The drawing under review shows one solid part. Ordinate dimensions are in mm from its lowest x, y, z. Coordinates: 2 decimals unless noted, no trailing zeros. Write each loop counter-clockwise with the first axis right and the second up, starting at its lowest first coordinate (ties: lowest second). Pieces come first, ordered by that corner, then holes. Notation, with made-up numbers: (-23, 88) - (-12, 88) arc R29 cw to (-12, 124) - close; hole circle Ø11 at (-34.5, -16.5). An arc over 180 degrees is marked (long way). Use a Markdown table: item, result.
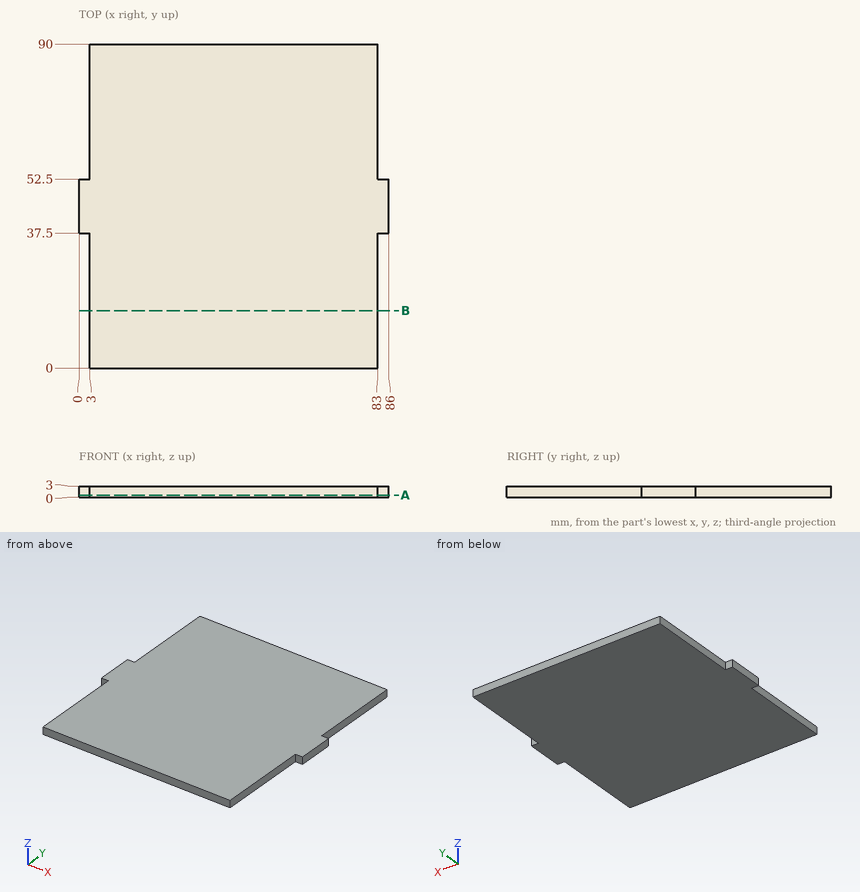
(1) Take a section at A-A on z = 0.55. Write out the cut boundary in (x, y), and give its area (3 significant figures).
Determined:
| item | result |
|---|---|
| outline | (0, 37.5) - (3, 37.5) - (3, 0) - (83, 0) - (83, 37.5) - (86, 37.5) - (86, 52.5) - (83, 52.5) - (83, 90) - (3, 90) - (3, 52.5) - (0, 52.5) - close |
| area | 7,290 mm2 |
(2) For L1, parallel to X at y = 18.5, z = 1.7, list the stretches that pass through material, from the lowest coordinate up. Write a range as from..to.
Determined:
| item | result |
|---|---|
| L1 | 3..83 |
(3) Take a section at B-B on y = 16. Write out the cut boundary in (x, z), and give its area (3 significant figures).
Determined:
| item | result |
|---|---|
| outline | (3, 0) - (83, 0) - (83, 3) - (3, 3) - close |
| area | 240 mm2 |
(4) For pin 1 (1.5 mm diameter, centred on x = 84, z = 1.5, fed in from +Y); pin 2 (0.9 mm diameter, centred on y = 76, z = 1.5, fed in from -X); pin 3 (1.5 mm diameter, centred on x = 2, z = 1.5, fed in from -Y), all flat-tipped, find the tip position at first contact; note any pin that passes through.
Determined:
| item | result |
|---|---|
| pin 1 | y = 52.5 |
| pin 2 | x = 3 |
| pin 3 | y = 37.5 |
